Build history of the part. All positions in model axes, mm. A direction names the side the tool comes from. Give positions to 0.01 mm unless a question says otherwise; leave off trailing zeros. Order: outer loops, then holes, each group sorted by start corner. A loop starts at its lowest first (then second) coordinate and runs counter-clockwise, first axis right, second up. Notation, with made-up numbers: M 18.25,58.25 L 43.25,58.25 A31 ccw 43.25,94.25 Z; hole C 2.5,8.25 d6. An arc over 180 degrees is marked long. One line per item, written item: value.
Autodesk Inventor part; units mm, degrees
ref_plane "YZ Plane" through (0, 0, 0) normal (1, 0, 0) x (0, 1, 0)
ref_plane "XZ Plane" through (0, 0, 0) normal (0, 1, 0) x (-1, 0, 0)
ref_plane "XY Plane" through (0, 0, 0) normal (0, 0, 1) x (1, 0, 0)
sketch "Sketch1" plane through (0, 0, 0) normal (0, 1, 0) x (-1, 0, 0)
  circle A0 centre (0, 0) radius 10
extrude "Extrusion1" add sketch "Sketch1" along normal blind 25
sketch "Sketch2" plane through (0, 0, 0) normal (0, 0, 1) x (1, 0, 0)
  line L0 (0, 0) -> (0, 12.7) construction
  circle A0 centre (0, 12.7) radius 6.5
extrude "Extrusion2" cut sketch "Sketch2" along normal through all both and the other way through all
sketch "Sketch3" plane through (0, 25, 0) normal (0, 1, 0) x (1, 0, 0)
  circle A0 centre (0, 0) radius 2
  dimension "d7" = 4
extrude "Extrusion3" cut sketch "Sketch3" against normal up to surface
fillet "Fillet1" radius 0.5 1 edges at (10, 25, 0)
properties part number "Cursore"
1) Saw through at B-B, the plane z = 0. Write the cut outline in (x, y).
Check values:
outline: M -10,0 L 10,0 L 10,24.5 A0.5 ccw 9.5,25 L 2,25 L 2,18.88 A6.5 cw long -2,18.88 L -2,25 L -9.5,25 A0.5 ccw -10,24.5 Z
2) Tool access for faces 4 (the face through (0, 22, 2)), 5 (the face through (0.1, 25, 2.2)): list every direction of +Z, -Z, +X, -X, +Y, -Y with a clear straight run to the whole face (end or side of a thin tool).
Check values:
face 4: +Y
face 5: +Z, -Z, +X, -X, +Y
3) Saw through at C-C, the plane y = 20.5. Write the cut outline in (x, z).
Check values:
outline: C 0,0 d20; hole C 0,0 d4
4) Saw through at A-A, the plane x = 0. Write the cut outline in (y, z), then the cut area to 3 significant figures.
Check values:
outline: M 0,-10 L 6.2,-10 L 6.2,10 L 0,10 Z; M 19.2,-10 L 24.5,-10 A0.5 ccw 25,-9.5 L 25,-2 L 19.2,-2 Z; M 19.2,2 L 25,2 L 25,9.5 A0.5 ccw 24.5,10 L 19.2,10 Z
area: 217 mm^2
5) Saw through at D-D, the plane y = 14. Write the cut outline in (x, z).
Check values:
outline: M -6.37,-7.71 L -6.37,7.71 A10 ccw Z; M 6.37,-7.71 A10 ccw 6.37,7.71 Z
6) Pin check, flat tips, straight feed: pin 1 (1.5 mm diameter, centred on x = 4.5, y = 9.5, fed in from +Z); pin 2 (5 mm diameter, centred on y = 2.5, z = -4.5, fed in from -X); pin 3 (8 mm diameter, centred on x = -2.5, y = 9.5, fed in from +Z). Stop position of each tip, or through.
Check values:
pin 1: through
pin 2: x = -9.8
pin 3: z = 10
7) Drill centre lines: probe 1 along Z at (x, y) = (0, 23.25); probe 2 along Y at (x, z) = (0, 5); probe 3 along Y at (x, z) = (-3, 6.5). Where is each one in solid material? Low to high. Write a range as from..to.
Check values:
probe 1: -10..-2, 2..10
probe 2: 0..6.2, 19.2..25
probe 3: 0..6.93, 18.47..25
8) Mould opens along X. For faces 1 (the face through (10, 12, 0)), 2 (the face through (0, 0, 0)), 3 (the face through (3.494, 7.219, -0.14)) say: released by +X, released by -X, zero draft, split by the parting line, or undercut.
Check values:
face 1: split by the parting line
face 2: zero draft
face 3: undercut
